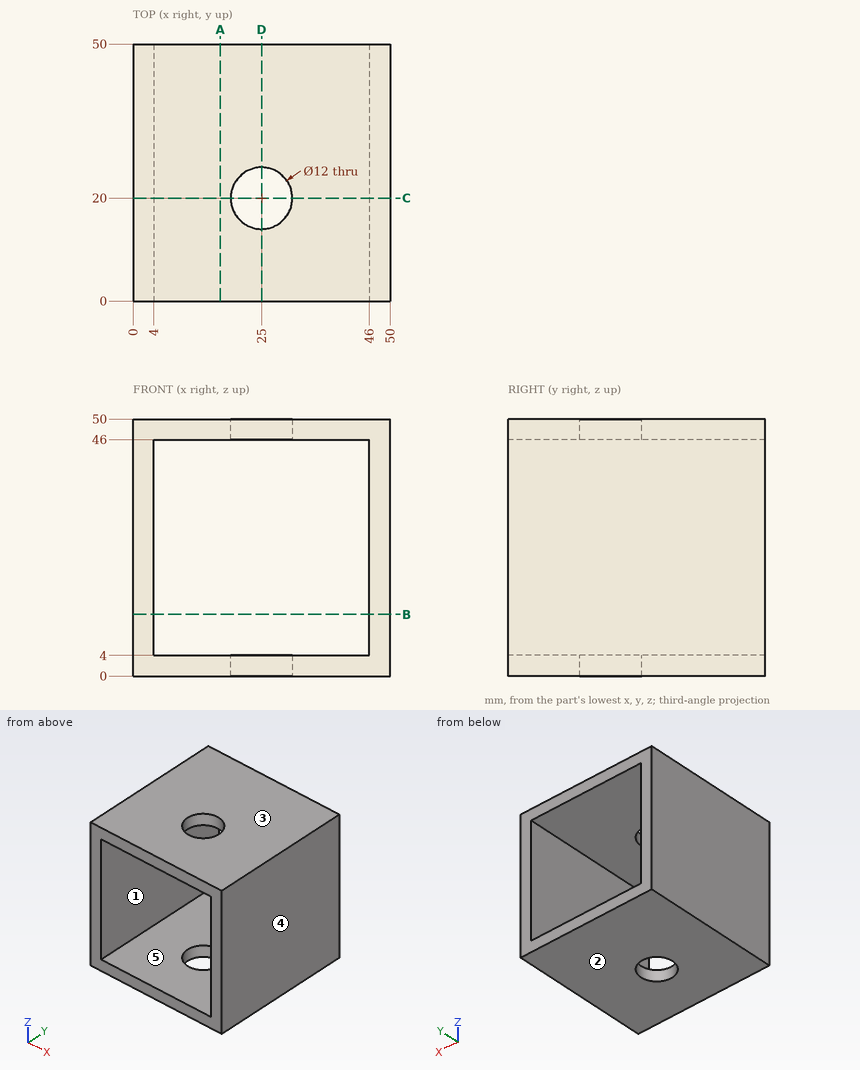
Input: dimensioned drawing with shaded views. Units: mm. Origin: part minimum x, y, z. A direction names the side the tool comes from. Give positions to 0.01 mm unless a question says otherwise; leave off trailing zeros. Write each loop counter-clockwise with the first axis right and the second up, starting at its lowest first coordinate (ties: lowest second). Pieces come first, ordered by that corner, then holes. Notation, with made-up numbers: M 34,-31 L 81,-31 A11 cw 81,-13 Z; hole C 60.5,-32.5 d9. An arc over 180 degrees is marked long. Return JSON: item names as keys, results as strings. Group by question number.
1) Cut plane C-C, the plane y = 20. Output: boundary loops of the cut face in (x, z), plus the area to 3 significant figures.
2) Set-up query: the marked faces 4 and 5. Return all of +Z, -Z, +X, -X, +Y, -Y with unobstructed straight access to the full face (end or side cutting, diameter ignored); none if empty.
3) Cut plane A-A, the plane x = 17. Output: boundary loops of the cut face in (y, z).
4) Material intervals for line 1 along Z through (x, y) = (35, 48); line 2 along Y through (x, z) = (25, 2.1), sorted ascending. Write a range as [from, to].
5) Cut plane B-B, the plane z = 12. Output: boundary loops of the cut face in (x, y), plus the area to 3 significant figures.
6) Pull-direction query (Z, two-part tool) for the marked faces 1, 2 and 3; classes: pulls with the +Z half, pulls with the -Z half, needs draft (parallel to the pull), parting line crosses it, or undercut.
7) Cut plane D-D, the plane x = 25. Output: boundary loops of the cut face in (y, z).
Recorded:
{
 "1": {"outline": "M 0,0 L 19,0 L 19,4 L 4,4 L 4,46 L 19,46 L 19,50 L 0,50 Z; M 31,0 L 50,0 L 50,50 L 31,50 L 31,46 L 46,46 L 46,4 L 31,4 Z", "area": "640 mm²"},
 "2": {"face 4": "+Z, -Z, +X, +Y, -Y", "face 5": "+Y, -Y"},
 "3": {"outline": "M 0,0 L 50,0 L 50,4 L 0,4 Z; M 0,46 L 50,46 L 50,50 L 0,50 Z"},
 "4": {"line 1": "z = [0, 4], [46, 50]", "line 2": "y = [0, 14], [26, 50]"},
 "5": {"outline": "M 0,0 L 4,0 L 4,50 L 0,50 Z; M 46,0 L 50,0 L 50,50 L 46,50 Z", "area": "400 mm²"},
 "6": {"face 1": "undercut", "face 2": "pulls with the -Z half", "face 3": "pulls with the +Z half"},
 "7": {"outline": "M 0,0 L 14,0 L 14,4 L 0,4 Z; M 0,46 L 14,46 L 14,50 L 0,50 Z; M 26,0 L 50,0 L 50,4 L 26,4 Z; M 26,46 L 50,46 L 50,50 L 26,50 Z"}
}
